Part model, mm, in its own coordinate system. Face numbers are marked on the shaded views. Round coordinates to 2 decimals unless told otherwise and drop trailing zeros. Write each loop counter-clockwise with the first axis right and the second up, starting at its lowest first coordinate (ties: lowest second). Pieces come first, ordered by that corner, then holes. Notation, with made-up numbers: (57, 39) -> (102, 39) arc R21 cw to (102, 67) -> close; hole circle Ø10 at (28, 33). An arc over 180 degrees is marked (long way). Return JSON: item names as keys, results as strings. Group by question number.
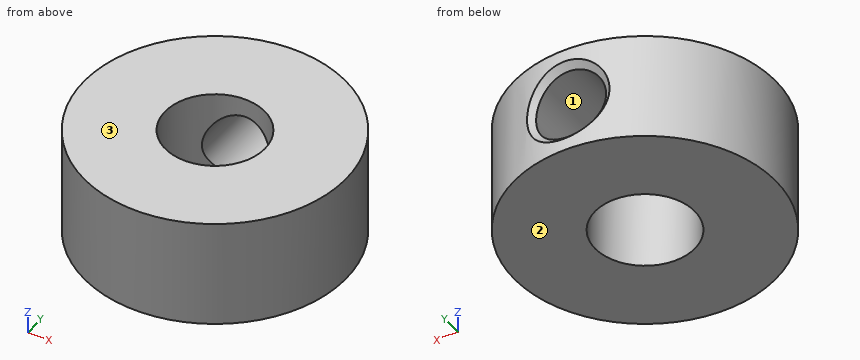
```python
from build123d import *

# Parameters (mm, degrees)
SKETCH_R     = 4
SKETCH_R_2   = 1.525
PAD_DEPTH    = 3.3
SKETCH001_R  = 1.075
HOLE_DEPTH   = 5
CHAMFER_SIZE = 0.2


with BuildPart() as part:
    # Sketch → Pad (new body)
    with BuildSketch(Plane.XY):
        Circle(SKETCH_R)
        Circle(SKETCH_R_2, mode=Mode.SUBTRACT)
    extrude(amount=PAD_DEPTH)

    # Sketch001 → Hole (cut)
    with BuildSketch(Plane.XZ):
        with Locations((0, 1.65)):
            Circle(SKETCH001_R)
    extrude(amount=-HOLE_DEPTH, mode=Mode.SUBTRACT)

    # Chamfer
    chamfer_edges = [part.edges().sort_by_distance(p)[0] for p in [
        (1.075, 3.85284, 1.65),
    ]]
    chamfer(chamfer_edges, length=CHAMFER_SIZE)


solid = part.part
```
Item 1: Two-plate mould, pull along Z, no slides. Class the marked faces 1, 2 and 3: released by +Z, released by -Z, zero draft, split by the parting line, or undercut.
Item 2: Flat gauge pins, fed straight in: P1, Ø1.9, axis at x = 0, z = 1.65, coming from the +Y side; P2, Ø1.5, axis at x = -0.5, z = 1.5, coming from the -Y side. Where does each tip first touch, or does it go through?
Item 3: Cut at D-D (x = -1.75). Write the cut outline in (y, z), then the cut area to 3 significant figures.
Item 4: Cut at C-C (y = -1.25). Write the cut outline in (x, z), then the cut area to 3 significant figures.
Item 5: Cut at A-A (y = 0). Write the cut outline in (x, z) (3 decimals), then the cut area to 3 significant figures.
Item 6: Wall check: L1, parallel to Z at x = 0, y = 1.8 (3 decimals); L2, parallel to X at y = 2.65, z = 1.65 (3 decimals); L3, parallel to X at y = 3, z = 1. Give the ranges that are in metal, low to high.
Checks:
{
 "1": {"face 1": "undercut", "face 2": "released by -Z", "face 3": "released by +Z"},
 "2": {"P1": "stops at y = -1.19", "P2": "stops at y = -4"},
 "3": {"outline": "(-3.6, 0) -> (3.6, 0) -> (3.6, 3.3) -> (-3.6, 3.3) -> close", "area": "23.7 mm2"},
 "4": {"outline": "(-3.8, 0) -> (-0.87, 0) -> (-0.87, 3.3) -> (-3.8, 3.3) -> close; (0.87, 0) -> (3.8, 0) -> (3.8, 3.3) -> (0.87, 3.3) -> close", "area": "19.3 mm2"},
 "5": {"outline": "(-4, 0) -> (-1.525, 0) -> (-1.525, 3.3) -> (-4, 3.3) -> close; (1.525, 0) -> (4, 0) -> (4, 3.3) -> (1.525, 3.3) -> close", "area": "16.3 mm2"},
 "6": {"L1": "z = 0 to 0.575, 2.725 to 3.3", "L2": "x = -2.996 to -1.075, 1.075 to 2.996", "L3": "x = -2.65 to -0.86, 0.86 to 2.65"}
}
